```python
from build123d import *

# Parameters (mm, degrees)
SKETCH1_W           = 65
SKETCH1_H           = 130
SKETCH1_R           = 1.5
BOSS_EXTRUDE1_DEPTH = 3
SKETCH2_R           = 1.5
CUT_EXTRUDE2_DEPTH  = 73.734104793
FILLET1_R           = 10


with BuildPart() as part:
    # Sketch1 → Boss-Extrude1 (new body)
    with BuildSketch(Plane(origin=(0, 0, 0), x_dir=(1, 0, 0), z_dir=(0, 1, 0))):
        Rectangle(SKETCH1_W, SKETCH1_H)
        with Locations(Location((-22.5, 22.5, 0), (0, 0, 270))):
            Circle(SKETCH1_R, mode=Mode.SUBTRACT)
        with Locations(Location((22.5, 22.5, 0), (0, 0, 270))):
            Circle(SKETCH1_R, mode=Mode.SUBTRACT)
        with Locations(Location((-22.5, -22.5, 0), (0, 0, 90))):
            Circle(SKETCH1_R, mode=Mode.SUBTRACT)
        with Locations(Location((22.5, -22.5, 0), (0, 0, 90))):
            Circle(SKETCH1_R, mode=Mode.SUBTRACT)
    extrude(amount=BOSS_EXTRUDE1_DEPTH)

    # Sketch2 → Cut-Extrude2 (cut, through all)
    with BuildSketch(Plane(origin=(0, 0, 0), x_dir=(1, 0, 0), z_dir=(0, 1, 0))):
        with Locations(Location((-12.5, 59, 0), (0, 0, 270))):
            Circle(SKETCH2_R)
        with Locations(Location((12.5, 59, 0), (0, 0, 270))):
            Circle(SKETCH2_R)
        with Locations(Location((12.5, 34, 0), (0, 0, 270))):
            Circle(SKETCH2_R)
        with Locations(Location((-12.5, 34, 0), (0, 0, 270))):
            Circle(SKETCH2_R)
    cut_extrude2 = extrude(amount=CUT_EXTRUDE2_DEPTH, mode=Mode.SUBTRACT)

    # Mirror1: Cut-Extrude2 across plane
    add(cut_extrude2.mirror(Plane.XY), mode=Mode.SUBTRACT)

    # Fillet1
    fillet1_edges = [part.edges().sort_by_distance(p)[0] for p in [
        (32.5, 1.5, -65),
        (32.5, 1.5, 65),
        (-32.5, 1.5, 65),
        (-32.5, 1.5, -65),
    ]]
    fillet(fillet1_edges, radius=FILLET1_R)


solid = part.part
```
Part model, mm, in its own coordinate system. Round coordinates to 2 decimals unless told otherwise and drop trailing zeros. Order: outer loops, then holes, each group sorted by start corner. A loop starts at its lowest first (then second) coordinate and runs counter-clockwise, first axis right, second up. Notation, with made-up numbers: M -38.5,23.25 L -11.5,23.25 A12 ccw -11.5,30.25 Z; hole C -18,-12.5 d6. An arc over 180 degrees is marked long. Answer in a Markdown table with one row per item. Add a question column.
Q1. Cut at D-D on z = -59. Give the cut face in (x, y).
Q2. Pin check, flat tip, straight feed: pin 1 (2.5 mm diameter, centred on x = -22.5, z = -22.5, fed in from +Y). Stop position of the tip, or through.
Q3. Cut at C-C on y = 0.6. Give the number of separate pieces and of enclosed holes in the cut face, and give its area (3 significant figures).
Q4. Mould opens along Z. For faces 1 (the face through (0, 3, -1)), 2 (the face through (12.95, 1.48, -57.57)), 3 (the face through (0, 1, 65)), 4 (the face through (29.49, 1.52, -62.15)) say: +Z half, -Z half, draft (parallel to the pull), parting line (faces both ways), or undercut.
Q5. Wall check: L1, parallel to X at y = 0.8, z = 22.5; L2, parallel to X at y = 0.6, z = 34; L3, parallel to Z at x = 12, y = 1.45. Give the ranges that are in metal, low to high. Write a range as from..to.
Q6. Cut at A-A on z = -22.5. Give the cut face in (x, y).
Q7. Cut at B-B on x = 12.5. Give the cut face in (y, z).
Established:
| question | item | result |
|---|---|---|
| 1 | outline | M -31.67,0 L -14,0 L -14,3 L -31.67,3 Z; M -11,0 L 11,0 L 11,3 L -11,3 Z; M 14,0 L 31.67,0 L 31.67,3 L 14,3 Z |
| 2 | pin 1 | passes through |
| 3 | separate pieces | 1 |
| 3 | enclosed holes | 12 |
| 3 | area | 8,280 mm2 |
| 4 | face 1 | draft |
| 4 | face 2 | undercut |
| 4 | face 3 | +Z half |
| 4 | face 4 | -Z half |
| 5 | L1 | x = -32.5..-24, -21..21, 24..32.5 |
| 5 | L2 | x = -32.5..-14, -11..11, 14..32.5 |
| 5 | L3 | z = -65..-60.41, -57.59..-35.41, -32.59..32.59, 35.41..57.59, 60.41..65 |
| 6 | outline | M -32.5,0 L -24,0 L -24,3 L -32.5,3 Z; M -21,0 L 21,0 L 21,3 L -21,3 Z; M 24,0 L 32.5,0 L 32.5,3 L 24,3 Z |
| 7 | outline | M 0,-65 L 3,-65 L 3,-60.5 L 0,-60.5 Z; M 0,-57.5 L 3,-57.5 L 3,-35.5 L 0,-35.5 Z; M 0,-32.5 L 3,-32.5 L 3,32.5 L 0,32.5 Z; M 0,35.5 L 3,35.5 L 3,57.5 L 0,57.5 Z; M 0,60.5 L 3,60.5 L 3,65 L 0,65 Z |
